```python
from build123d import *

# Parameters (mm, degrees)
EXTRUDE_1_DEPTH         = 150
FILLET_1_R              = 10
CUT_EXTRUDE_1_DEPTH     = 309.058436015
SKETCH1_R               = 12.5
CUT_EXTRUDE1_DEPTH      = 10
CUT_EXTRUDE2_DEPTH      = 80
CUT_EXTRUDE2_DEPTH_BACK = 10
SKETCH2_R               = 5
SKETCH4_R               = 12.5
SKETCH4_R_2             = 11.405
BOSS_EXTRUDE1_DEPTH     = 10
SKETCH8_R               = 5
BOSS_EXTRUDE3_DEPTH     = 90
SKETCH9_R               = 7
SKETCH9_R_2             = 5
BOSS_EXTRUDE4_DEPTH     = 3.5
BOSS_EXTRUDE5_START     = 3.5
SKETCH10_R              = 7
SKETCH10_R_2            = 5
BOSS_EXTRUDE5_DEPTH     = 3.5


with BuildPart() as part:
    # 草圖1 → 填料-伸長1 (new body)
    with BuildSketch(Plane(origin=(0, 0, 0), x_dir=(0, 0, -1), z_dir=(1, 0, 0))):
        with BuildLine():
            Line((0, 0), (0, 160))
            ThreePointArc((0, 160), (-21.611444176, 195.522683101), (-63.093050736, 192.660542061))
            Line((-63.093050736, 192.660542061), (-180, 110))
            Line((-180, 110), (-180, 0))
            Line((-180, 0), (0, 0))
        make_face()
    extrude(amount=EXTRUDE_1_DEPTH)

    # 圓角1
    fillet_1_edges = [part.edges().sort_by_distance(p)[0] for p in [
        (75, 110, 180),
    ]]
    fillet(fillet_1_edges, radius=FILLET_1_R)

    # 草圖2 → 除料-伸長1 (cut, through all)
    with BuildSketch(Plane(origin=(0, 0, 0), x_dir=(-1, 0, 0), z_dir=(0, 0, -1))):
        Polygon((-150, 110), (-125, 200), (-125, 212.317241835), (-176.077029544, 212.317241835), (-176.077029544, 111.407234288), align=None)
        Polygon((-110, 110), (-110, 202.916849344), (-40, 202.916849344), (-40, 110), (-40, 100), (-110, 100), align=None)
        Polygon((26.077029544, 111.407234288), (0, 110), (-25, 200), (-25, 212.317241835), (26.077029544, 212.317241835), align=None)
    extrude(amount=-CUT_EXTRUDE_1_DEPTH, mode=Mode.SUBTRACT)

    # Sketch1 → Cut-Extrude1 (cut)
    with BuildSketch(Plane.XZ):
        with Locations(Location((75, 40, 0), (0, 0, 270))):
            Circle(SKETCH1_R)
    extrude(amount=-CUT_EXTRUDE1_DEPTH, mode=Mode.SUBTRACT)

    # Sketch2 → Cut-Extrude2 (cut, two sides: drawn at the far end of the back side and taken through both)
    with BuildSketch(Plane(origin=(40, 0, 0), x_dir=(0, 0, -1), z_dir=(1, 0, 0)).offset(-CUT_EXTRUDE2_DEPTH_BACK)):
        with Locations(Location((-40, 160, 0), (0, 0, 270))):
            Circle(SKETCH2_R)
    extrude(amount=CUT_EXTRUDE2_DEPTH + CUT_EXTRUDE2_DEPTH_BACK, mode=Mode.SUBTRACT)

    # Sketch4 → Boss-Extrude1 (add)
    with BuildSketch(Plane.XZ):
        with Locations((75, 40)):
            Circle(SKETCH4_R)
        with Locations(Location((75, 40, 0), (0, 0, 270))):
            Circle(SKETCH4_R_2, mode=Mode.SUBTRACT)
    extrude(amount=-BOSS_EXTRUDE1_DEPTH)

    # Sketch8 → Boss-Extrude3 (add)
    with BuildSketch(Plane.ZY.offset(-120)):
        with Locations(Location((40, 160, 0), (0, 0, 90))):
            Circle(SKETCH8_R)
    extrude(amount=BOSS_EXTRUDE3_DEPTH)

    # Sketch9 → Boss-Extrude4 (add)
    with BuildSketch(Plane.ZY.offset(-110)):
        with Locations(Location((40, 160, 0), (0, 0, 180))):
            Circle(SKETCH9_R)
        with Locations((40, 160)):
            Circle(SKETCH9_R_2, mode=Mode.SUBTRACT)
    extrude(amount=BOSS_EXTRUDE4_DEPTH)

    # Sketch10 → Boss-Extrude5 (add)
    with BuildSketch(Plane(origin=(40, 0, 0), x_dir=(0, 0, -1), z_dir=(1, 0, 0)).offset(BOSS_EXTRUDE5_START)):
        with Locations((-40, 160)):
            Circle(SKETCH10_R)
        with Locations(Location((-40, 160, 0), (0, 0, 90))):
            Circle(SKETCH10_R_2, mode=Mode.SUBTRACT)
    extrude(amount=-BOSS_EXTRUDE5_DEPTH)


solid = part.part
```
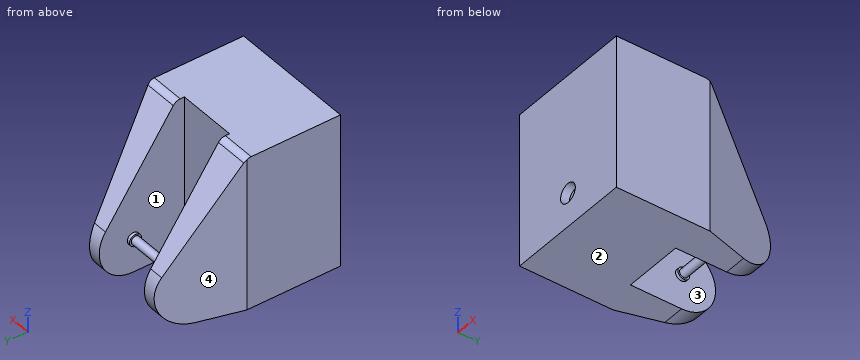
Design review of the part built by this model. Coordinates are the model's own, in mm. Face numbers are marked on the shaded views. Round coordinates to 2 decimals unless told otherwise and drop trailing zeros. Write each loop counter-clockwise with the first axis right and the second up, starting at its lowest first coordinate (ties: lowest second). Pieces come first, ordered by that corner, then holes. Notation, with made-up numbers: (15.25, 25) -> (20.25, 25) arc R30 cw to (20.25, 56) -> close; hole circle Ø6 at (-29.75, 67.25). An arc over 180 degrees is marked (long way). Answer in a Markdown table with one row per item.
Q1. Draft analysis for pull direction X (two halves, no side actions). For the marked faces 1, 2, 3 and 4, state which applies: +X half, -X half, draft (parallel to the pull), parting line (faces both ways), or undercut.
The answers:
| item | result |
|---|---|
| face 1 | undercut |
| face 2 | draft |
| face 3 | undercut |
| face 4 | -X half |
Q2. Take a section at A-A, the plane z = 40. State the section outline as (x, y) points (3 decimals), then the cut area to 3 significant figures.
The answers:
| item | result |
|---|---|
| outline | (0, 0) -> (63.595, 0) -> (63.595, 10) -> (86.405, 10) -> (86.405, 0) -> (150, 0) -> (150, 110) -> (125, 200) -> (110, 200) -> (110, 167) -> (106.5, 167) -> (106.5, 165) -> (43.5, 165) -> (43.5, 167) -> (40, 167) -> (40, 200) -> (25, 200) -> (0, 110) -> close; hole (40, 100) -> (110, 100) -> (110, 153) -> (106.5, 153) -> (106.5, 155) -> (43.5, 155) -> (43.5, 153) -> (40, 153) -> close |
| area | 21,200 mm² |
Q3. Clearance check with flat-ended pins moving along their axes: pin 1 Ø21 at (x, z) = (79.5, 120) entering from +Y; pin 2 Ø10 at (y, z) = (146.5, 63.5) entering from -X; pin 3 Ø7 at (y, z) = (159.5, 37) entering from +X; pin 4 Ø4 at (y, z) = (56.5, 34) entering from -X. State where each tip first meets the part, or that it passes through.
The answers:
| item | result |
|---|---|
| pin 1 | y = 100 |
| pin 2 | x = 8.75 |
| pin 3 | x = 137.22 |
| pin 4 | x = 0 |
Q4. Take a section at C-C, the plane x = 34. State the section outline as (y, z) points.
The answers:
| item | result |
|---|---|
| outline | (0, 0) -> (160, 0) arc R40 ccw to (192.66, 63.09) -> (112.99, 175.77) arc R10 ccw to (104.82, 180) -> (0, 180) -> close |
Q5. To check wall thickness, follow L1, parallel to X at y = 109, z = 69; L2, parallel to X at y = 5, z = 40 (3 decimals); L3, parallel to Y at x = 47.5, z = 54.5. State the ranges of each line that lie inside material, in increasing order. Write a range as [from, to].
The answers:
| item | result |
|---|---|
| L1 | [0, 40], [110, 150] |
| L2 | [0, 63.595], [86.405, 150] |
| L3 | [0, 100] |
Q6. Take a section at B-B, the plane x = 75. State the section outline as (y, z) points (3 decimals).
The answers:
| item | result |
|---|---|
| outline | (0, 0) -> (100, 0) -> (100, 180) -> (0, 180) -> (0, 51.405) -> (10, 51.405) -> (10, 28.595) -> (0, 28.595) -> close; circle Ø10 at (160, 40) |
Q7. Take a section at D-D, the plane y = 185.5. State the section outline as (x, z) points.
The answers:
| item | result |
|---|---|
| outline | (20.97, 9.18) -> (40, 9.18) -> (40, 73.22) -> (20.97, 73.22) -> close; (110, 9.18) -> (129.03, 9.18) -> (129.03, 73.22) -> (110, 73.22) -> close |
